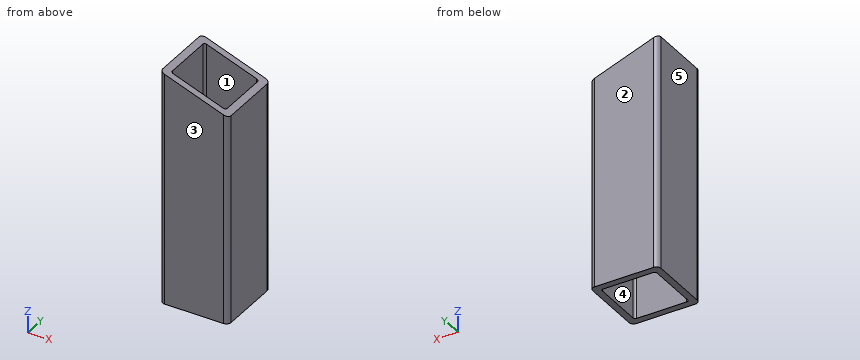
```python
from build123d import *

# Parameters (mm, degrees)
DODANIE_WYCI_GNI_CIE1_DEPTH = 103
WYTNIJ_WYCI_GNI_CIE1_DEPTH  = 70


with BuildPart() as part:
    # Szkic1 → Dodanie-wyciągnięcie1 (new body)
    with BuildSketch(Plane.XY):
        with BuildLine():
            Line((-13, -3), (13, -3))
            ThreePointArc((13, -3), (14.414213562, -2.414213562), (15, -1))
            Line((15, -1), (15, 25))
            ThreePointArc((15, 25), (14.414213562, 26.414213562), (13, 27))
            Line((13, 27), (-13, 27))
            ThreePointArc((-13, 27), (-14.414213562, 26.414213562), (-15, 25))
            Line((-15, 25), (-15, -1))
            ThreePointArc((-15, -1), (-14.414213562, -2.414213562), (-13, -3))
        make_face()
        with BuildLine():
            Line((-11, 0), (11, 0))
            ThreePointArc((11, 0), (11.707106781, 0.292893219), (12, 1))
            Line((12, 1), (12, 23))
            ThreePointArc((12, 23), (11.707106781, 23.707106781), (11, 24))
            Line((11, 24), (-11, 24))
            ThreePointArc((-11, 24), (-11.707106781, 23.707106781), (-12, 23))
            Line((-12, 23), (-12, 1))
            ThreePointArc((-12, 1), (-11.707106781, 0.292893219), (-11, 0))
        make_face(mode=Mode.SUBTRACT)
    extrude(amount=DODANIE_WYCI_GNI_CIE1_DEPTH)

    # Szkic2 → Wytnij-wyciągnięcie1 (cut)
    with BuildSketch(Plane.XZ.offset(3)):
        Polygon((-15, 103), (66.156264481, 73.461535405), (66.156264481, 103), align=None)
    extrude(amount=-WYTNIJ_WYCI_GNI_CIE1_DEPTH, mode=Mode.SUBTRACT)


solid = part.part
```
Design review of the part built by this model. Coordinates are the model's own, in mm. Face numbers are marked on the shaded views. A direction names the side the tool comes from. Round coordinates to 2 decimals unless told otherwise and drop trailing zeros. Order: outer loops, then holes, each group sorted by start corner. A loop starts at its lowest first (then second) coordinate and runs counter-clockwise, first axis right, second up. Notation, with made-up numbers: M -9,11.5 L -5,11.5 A13 ccw -5,27.5 Z; hole C 75.5,76.25 d2. An arc over 180 degrees is marked long. Put each result on its own line as item: value.
Q1. Insertion check: pin 1 Ø12 at (x, y) = (-8.5, 3.5) entering from +Z. The pin has a flat end and moves straight along its axis. Give the tip position at first contact, or say it passes through.
Reported:
pin 1: z = 102.82
Q2. To check wall thickness, follow line 1 (Y direction, x = 6.5, z = 81); line 2 (X direction, y = 7, z = 67.5); line 3 (X direction, y = 20.25, z = 97). State the ranges of each line that lie inside material, in increasing order.
Reported:
line 1: -3 to 0, 24 to 27
line 2: -15 to -12, 12 to 15
line 3: -15 to -12
Q3. Consider section B-B (z = 60). State the section outline as (x, y) points, and give its area (3 significant figures).
Reported:
outline: M -15,-1 A2 ccw -13,-3 L 13,-3 A2 ccw 15,-1 L 15,25 A2 ccw 13,27 L -13,27 A2 ccw -15,25 Z; hole M -12,1 A1 ccw -11,0 L 11,0 A1 ccw 12,1 L 12,23 A1 ccw 11,24 L -11,24 A1 ccw -12,23 Z
area: 321 mm²
Q4. Consider section C-C (x = 1.25). State the section outline as (y, z) points, and give its area (3 significant figures).
Reported:
outline: M -3,0 L 0,0 L 0,97.09 L -3,97.09 Z; M 24,0 L 27,0 L 27,97.09 L 24,97.09 Z
area: 583 mm²
Q5. Draft analysis for pull direction Y (two halves, no side actions). For the marked faces 3, 4 and 5, state which applies: released by +Y, released by -Y, zero draft, split by the parting line, or undercut.
Reported:
face 3: released by -Y
face 4: undercut
face 5: zero draft
Q6. Consider section A-A (y = 18). State the section outline as (x, z) points.
Reported:
outline: M -15,0 L -12,0 L -12,101.91 L -15,103 Z; M 12,0 L 15,0 L 15,92.08 L 12,93.17 Z
Q7. Machinability: for the marked faces 1 and 2, which of the approach directions +Z, -Z, +X, -X, +Y, -Y give a long, thin tool a straight path to every point of the face, cutting with its end or side? Answer none if there is none.
Reported:
face 1: +Z, -Z
face 2: +Z, -Z, +X, -X, +Y
